Here's the drawing with two shaded views (mm, measured from the low corner). I have some questions. Round coordinates to 2 decimals unless told otherwise and drop trailing zeros. Write each loop counter-clockwise with the first axis right and the second up, starting at its lowest first coordinate (ties: lowest second). Pieces come first, ordered by that corner, then holes. Notation, with made-up numbers: M -23.5,86.25 L 17.5,86.25 A21 ccw 17.5,113.25 Z; hole C 49,32 d2. An arc over 180 degrees is marked long. Answer as a JSON object with one key per item and string values. Group by question number.
1) Suppose I cut it at A-A, the plane x = 27.5. Write out the boundary of the cut face in (y, z), and give its area (3 significant figures).
2) Please list where these lines run through material, in increasing order: L1, parallel to Z at x = 105.5, y = 2.9; L2, parallel to Z at x = 27.5, y = 2.15; L3, parallel to X at y = 2.55, z = 11. Write a range as [from, to].
3) Suppose I cut it at D-D, the plane x = 105. Write out the boundary of the cut face in (y, z), and give its area (3 significant figures).
4) Suppose I cut it at B-B, the plane z = 10. Write out the boundary of the cut face in (x, y), and give its area (4 significant figures).
5) Suppose I cut it at C-C, the plane z = 4. Write out the boundary of the cut face in (x, y), and give its area (4 significant figures).
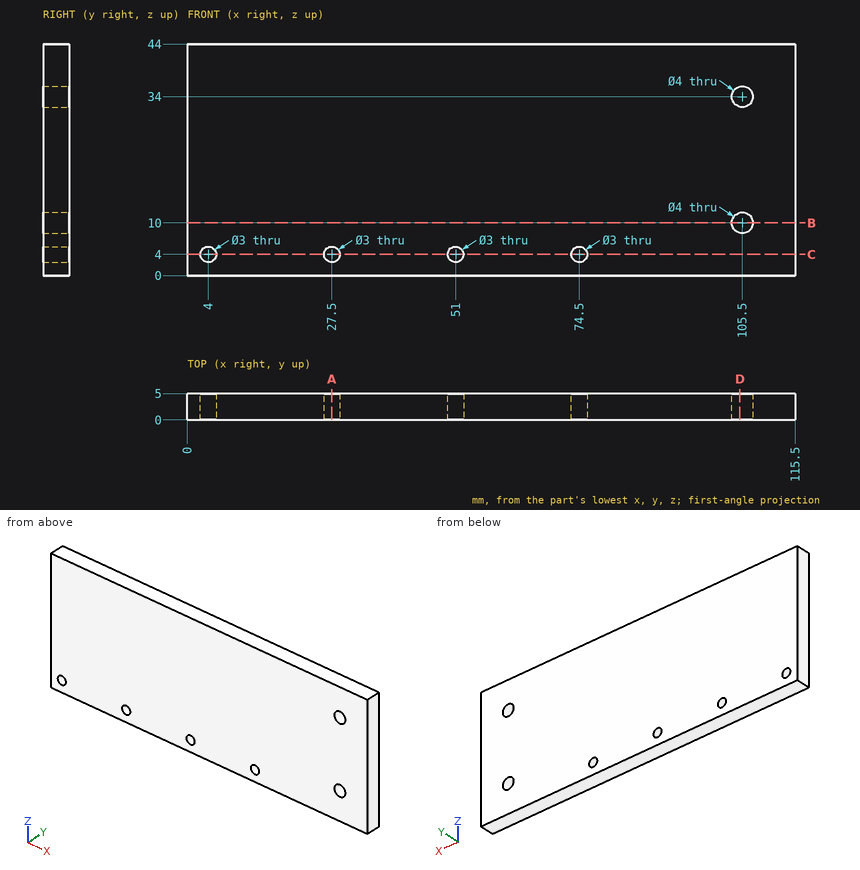
Results:
{
 "1": {"outline": "M 0,0 L 5,0 L 5,2.5 L 0,2.5 Z; M 0,5.5 L 5,5.5 L 5,44 L 0,44 Z", "area": "205 mm^2"},
 "2": {"L1": "[0, 8], [12, 32], [36, 44]", "L2": "[0, 2.5], [5.5, 44]", "L3": "[0, 103.77], [107.23, 115.5]"},
 "3": {"outline": "M 0,0 L 5,0 L 5,8.06 L 0,8.06 Z; M 0,11.94 L 5,11.94 L 5,32.06 L 0,32.06 Z; M 0,35.94 L 5,35.94 L 5,44 L 0,44 Z", "area": "181 mm^2"},
 "4": {"outline": "M 0,0 L 103.5,0 L 103.5,5 L 0,5 Z; M 107.5,0 L 115.5,0 L 115.5,5 L 107.5,5 Z", "area": "557.5 mm^2"},
 "5": {"outline": "M 0,0 L 2.5,0 L 2.5,5 L 0,5 Z; M 5.5,0 L 26,0 L 26,5 L 5.5,5 Z; M 29,0 L 49.5,0 L 49.5,5 L 29,5 Z; M 52.5,0 L 73,0 L 73,5 L 52.5,5 Z; M 76,0 L 115.5,0 L 115.5,5 L 76,5 Z", "area": "517.5 mm^2"}
}
